```python
from build123d import *

# Parameters (mm, degrees)
F1_DEPTH = 600
F2_T     = -25
F3_DEPTH = 12.5
F4_W     = 500
F4_H     = 1150
F5_DEPTH = 12.5
F7_W     = 1150
F7_H     = 350
F8_DEPTH = 12.5
F10_D    = 10


with BuildPart() as f1:
    # F0 (on Front) → F1 (new body, symmetric)
    with BuildSketch(Plane.XZ):
        Polygon((0, 200), (-400, 200), (-600, -200), (0, -200), align=None)
    extrude(amount=F1_DEPTH, both=True)

    # F2
    f2_openings = [f1.faces().sort_by_distance(p)[0] for p in [
        (0, 0, 0),
        (-500, 0, 0),
    ]]
    offset(amount=F2_T, openings=f2_openings)

    # F0 (on Front) → F3 (join, symmetric)
    with BuildSketch(Plane.XZ):
        Polygon((0, 200), (-400, 200), (-600, -200), (0, -200), align=None)
    extrude(amount=F3_DEPTH, both=True)

    # F4 (on Top) → F5 (join, symmetric)
    with BuildSketch(Plane.XY):
        with Locations((-250, 0)):
            Rectangle(F4_W, F4_H)
    extrude(amount=F5_DEPTH, both=True)

    # F7 (on offset) → F8 (join, symmetric)
    with BuildSketch(Plane.YZ.offset(-300)):
        Rectangle(F7_W, F7_H)
    extrude(amount=F8_DEPTH, both=True)

    # F10 (through all)
    with Locations(Plane(origin=(0, 0, -200), x_dir=(1, 0, 0), z_dir=(0, 0, -1))):
        with Locations((-40, 560), (-547.5, 560), (-40, -560), (-547.5, -560), (-360, 560), (-360, -560)):
            Hole(F10_D / 2)


solid = f1.part
```
Geometry check sheet. Reference: the model listing, model coordinates, mm. A direction names the side the tool comes from. Coordinates: 2 decimals unless noted, no trailing zeros. Order: outer loops, then holes, each group sorted by start corner. A loop starts at its lowest first (then second) coordinate and runs counter-clockwise, first axis right, second up. Notation, with made-up numbers: M -33,0 L 13,0 A20 cw 13,4 Z; hole C 66.5,43 d7. An arc over 180 degrees is marked long. One line per question, with ' | ' between items. Start each with the question number.
Item 1: Cross-section at A-A on z = -35. Enter the section's corners in (x, y).
Item 2: Material ranges on L1, parallel to Z at x = -392, y = -75.5; L2, parallel to X at y = -560, z = -3; L3, parallel to Y at x = -115, z = 131.5, recorded low to high. Write a range as [from, to].
Item 3: Draft check along Y on faces 4 (the flat face through (-421, 575, -106)), 5 (the flat face through (-238, 600, 3)), 6 (the flat face through (-146, -298, -175)), 7 (the flat face through (-304, -8, -200)). Enter one of: pulls with the +Y half, pulls with the -Y half, needs draft (parallel to the pull), parting line crosses it, or undercut.
Item 4: Cross-section at C-C on y = -145. Enter the section's corners in (x, z).
Item 5: Cross-section at B-B on x = -253.5. Enter the section's corners in (y, z).
Item 6: Set-up check for faces 1 (the flat face through (-384, 12.5, 95)), 2 (the flat face through (0, -47, -1)), 3 (the flat face through (-146, 290, -175)): record each of +Z, -Z, +X, -X, +Y, -Y from which the full face is reachable in a straight line by a thin tool's end or side.
Item 7: Gauge pin test, flat ends, axial feed: pin 1 (12 mm diameter, centred on y = 241, z = -149, fed in from -X); pin 2 (6 mm diameter, centred on x = -547.5, y = -560, fed in from +Z); pin 3 (13 mm diameter, centred on x = -360, y = 560, fed in from -Z); pin 4 (12 mm diameter, centred on x = -510, y = 350.5, fed in from +Z). Record the tip position at first contact, or that the pin passes through.
Findings:
1) outline: M -517.5,-600 L 0,-600 L 0,-575 L -287.5,-575 L -287.5,-12.5 L 0,-12.5 L 0,12.5 L -287.5,12.5 L -287.5,575 L 0,575 L 0,600 L -517.5,600 L -517.5,575 L -312.5,575 L -312.5,12.5 L -517.5,12.5 L -517.5,-12.5 L -312.5,-12.5 L -312.5,-575 L -517.5,-575 Z
2) L1: z = [-200, -175], [-12.5, 12.5], [175, 200] | L2: x = [-500, -365], [-355, -45], [-35, 0] | L3: y = [-600, -575], [-12.5, 12.5], [575, 600]
3) face 4: undercut | face 5: pulls with the +Y half | face 6: undercut | face 7: needs draft
4) outline: M -600,-200 L 0,-200 L 0,-175 L -287.5,-175 L -287.5,-12.5 L 0,-12.5 L 0,12.5 L -287.5,12.5 L -287.5,175 L 0,175 L 0,200 L -400,200 L -412.5,175 L -312.5,175 L -312.5,12.5 L -500,12.5 L -500,-12.5 L -312.5,-12.5 L -312.5,-175 L -587.5,-175 Z
5) outline: M -600,-200 L 600,-200 L 600,200 L -600,200 Z; hole M -575,-175 L -12.5,-175 L -12.5,-12.5 L -575,-12.5 Z; hole M -575,12.5 L -12.5,12.5 L -12.5,175 L -575,175 Z; hole M 12.5,-175 L 575,-175 L 575,-12.5 L 12.5,-12.5 Z; hole M 12.5,12.5 L 575,12.5 L 575,175 L 12.5,175 Z
6) face 1: -X | face 2: +Z, -Z, +X, +Y, -Y | face 3: +X
7) pin 1: stops at x = -312.5 | pin 2: passes through | pin 3: stops at z = -200 | pin 4: stops at z = -175
